from build123d import *

# Parameters (mm, degrees)
SKETCH1_R           = 1.7
SKETCH1_R_2         = 1.5875
SKETCH1_W           = 4
SKETCH1_H           = 12
SKETCH1_W_2         = 12
SKETCH1_H_2         = 4
SKETCH1_W_3         = 6
SKETCH1_H_3         = 8
BOSS_EXTRUDE2_DEPTH = 6


with BuildPart() as part:
    # Sketch1 → Boss-Extrude2 (new body)
    with BuildSketch(Plane(origin=(0, 0, 0), x_dir=(1, 0, 0), z_dir=(0, 1, 0))):
        with BuildLine():
            Line((90, 80), (-20, 80))
            ThreePointArc((-20, 80), (-27.071067812, 77.071067812), (-30, 70))
            Line((-30, 70), (-30, -75))
            ThreePointArc((-30, -75), (-27.071067812, -82.071067812), (-20, -85))
            Line((-20, -85), (90, -85))
            ThreePointArc((90, -85), (97.071067812, -82.071067812), (100, -75))
            Line((100, -75), (100, 70))
            ThreePointArc((100, 70), (97.071067812, 77.071067812), (90, 80))
        make_face()
        with Locations(Location((41.804775222, 18, 0), (0, 0, 270))):
            Circle(SKETCH1_R, mode=Mode.SUBTRACT)
        with Locations(Location((78.304775222, 17.96923253, 0), (0, 0, 270))):
            Circle(SKETCH1_R, mode=Mode.SUBTRACT)
        with Locations(Location((78.304775222, -18.53076747, 0), (0, 0, 270))):
            Circle(SKETCH1_R, mode=Mode.SUBTRACT)
        with Locations(Location((41.804775222, -18.5, 0), (0, 0, 270))):
            Circle(SKETCH1_R, mode=Mode.SUBTRACT)
        with Locations(Location((39.806499109, -29.593870337, 0), (0, 0, 270))):
            Circle(SKETCH1_R_2, mode=Mode.SUBTRACT)
        with Locations(Location((91.876499109, -34.673870337, 0), (0, 0, 270))):
            Circle(SKETCH1_R_2, mode=Mode.SUBTRACT)
        with Locations(Location((91.876499109, -62.613870337, 0), (0, 0, 270))):
            Circle(SKETCH1_R_2, mode=Mode.SUBTRACT)
        with Locations(Location((41.076499109, -77.853870337, 0), (0, 0, 270))):
            Circle(SKETCH1_R_2, mode=Mode.SUBTRACT)
        with Locations((-17, 0)):
            Rectangle(SKETCH1_W, SKETCH1_H, mode=Mode.SUBTRACT)
        with Locations((0, 17)):
            Rectangle(SKETCH1_W_2, SKETCH1_H_2, mode=Mode.SUBTRACT)
        with Locations((17, 0)):
            Rectangle(SKETCH1_W, SKETCH1_H, mode=Mode.SUBTRACT)
        with Locations((0, -17)):
            Rectangle(SKETCH1_W_2, SKETCH1_H_2, mode=Mode.SUBTRACT)
        with Locations((23.479105259, 66.763598247)):
            Rectangle(SKETCH1_W_3, SKETCH1_H_3, mode=Mode.SUBTRACT)
        with Locations((49.479105259, 66.763598247)):
            Rectangle(SKETCH1_W_3, SKETCH1_H_3, mode=Mode.SUBTRACT)
    extrude(amount=BOSS_EXTRUDE2_DEPTH)


solid = part.part
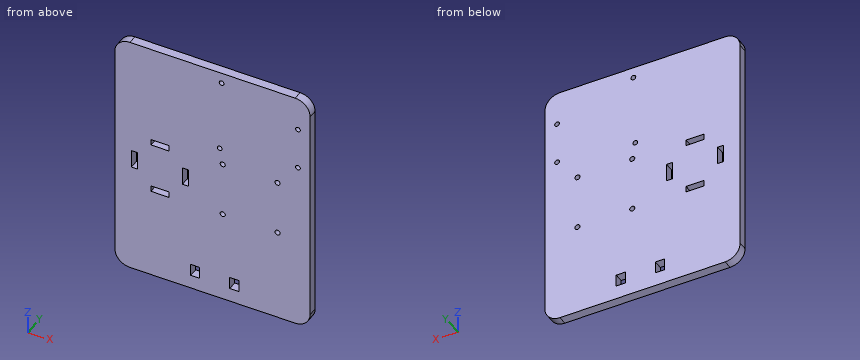
Input: part model. Units: mm. Frame: model coordinates. Round coordinates to 2 decimals unless told otherwise and drop trailing zeros. Loops run counter-clockwise (first coordinate to the right, second up) from the corner with the lowest first, then second, coordinate; pieces in that order, holes last. Notation, with made-up numbers: (76, -0.75) -> (121, -0.75) arc R19 cw to (121, 8.25) -> close; hole circle Ø6 at (65, 58.5). An arc over 180 degrees is marked (long way). Answer as a JSON object with one key per item and string values. Group by question number.
1) Section query A-A on z = 0. Output: boundary loops of the cut face in (x, y), plus the area to 3 significant figures.
2) Section query B-B on y = 3.95. State how many separate pieces and enclosed holes the cut face has, plus the area to 3 significant figures.
3) Ray query, L1, parallel to Z at x = 1, y = 4.2; L2, parallel to X at y = 3.2, z = -18; L3, parallel to X at y = 4.55, z = -65. Return the intervals inside material, ascending.
4) Pin query (flat end, axial travel): pin 1 (3 mm diameter, centred on x = 78.3, z = 18.53, fed in from -Y). Return the tip coordinate at first contact, or that it passes through.
Reply:
{
 "1": {"outline": "(-30, 0) -> (-19, 0) -> (-19, 6) -> (-30, 6) -> close; (-15, 0) -> (15, 0) -> (15, 6) -> (-15, 6) -> close; (19, 0) -> (100, 0) -> (100, 6) -> (19, 6) -> close", "area": "732 mm2"},
 "2": {"separate pieces": "1", "enclosed holes": "14", "area": "21,000 mm2"},
 "3": {"L1": "z = -80 to -19, -15 to 15, 19 to 85", "L2": "x = -30 to -6, 6 to 40.1, 43.5 to 76.61, 80 to 100", "L3": "x = -30 to 20.48, 26.48 to 46.48, 52.48 to 100"},
 "4": {"pin 1": "passes through"}
}
